Input: part model. Units: mm. Frame: model coordinates. Face numbers are marked on the shaded views. A direction names the side the tool comes from. Give positions to 0.01 mm unless a question says otherwise; leave off trailing zeros. Loops run counter-clockwise (first coordinate to the right, second up) from the corner with the lowest first, then second, coordinate; pieces in that order, holes last. Notation, with made-up numbers: (71, 62.25) -> (76, 62.25) arc R31 cw to (76, 97.25) -> close; hole circle Ø1 at (-2.5, -37.5). An arc over 180 degrees is marked (long way). Use CSV: the item, a comma, the result in double quotes.
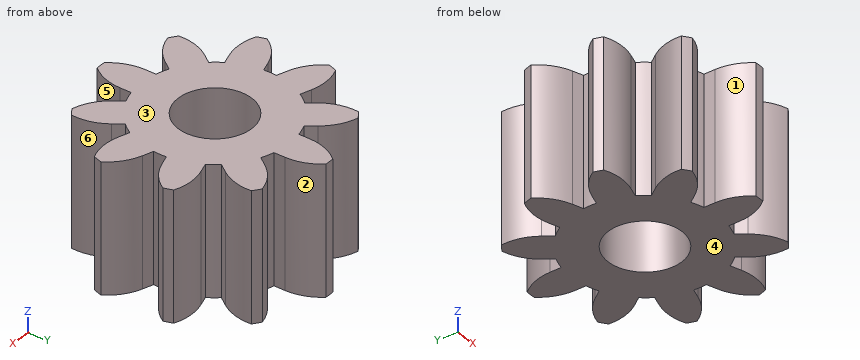
```python
from build123d import *

# Parameters (mm, degrees)
ESBO_O1_R                = 2
RESSALTO_EXTRUS_O1_DEPTH = 3.5
CORTE_EXTRUS_O1_REACH    = 7.574
ESBO_O2_R                = 1


with BuildPart() as part:
    # Esboço1 → Ressalto-extrusão1 (new body)
    with BuildSketch(Plane.XY):
        Circle(ESBO_O1_R)
        with BuildLine():
            Line((-1.99959981, -1.122867364), (-1.714282855, -1.030162265))
            ThreePointArc((-1.714282855, -1.030162265), (-1.902113033, -0.618033989), (-1.99239815, -0.174211401))
            Line((-1.99239815, -0.174211401), (-2.277715105, -0.266916499))
            ThreePointArc((-2.277715105, -0.266916499), (-2.695113044, -0.490735084), (-3.008300145, -0.846023191))
            ThreePointArc((-3.008300145, -0.846023191), (-2.972051613, -0.965678107), (-2.931045896, -1.08378732))
            ThreePointArc((-2.931045896, -1.08378732), (-2.4688391, -1.187134677), (-1.99959981, -1.122867364))
        make_face()
        with BuildLine():
            Line((-2.277715105, 0.266916499), (-1.99239815, 0.174211401))
            ThreePointArc((-1.99239815, 0.174211401), (-1.902113033, 0.618033989), (-1.714282855, 1.030162265))
            Line((-1.714282855, 1.030162265), (-1.99959981, 1.122867364))
            ThreePointArc((-1.99959981, 1.122867364), (-2.4688391, 1.187134677), (-2.931045896, 1.08378732))
            ThreePointArc((-2.931045896, 1.08378732), (-2.972051613, 0.965678107), (-3.008300145, 0.846023191))
            ThreePointArc((-3.008300145, 0.846023191), (-2.695113044, 0.490735084), (-2.277715105, 0.266916499))
        make_face()
        with BuildLine():
            Line((-1.685820646, 1.554747331), (-1.509485071, 1.312042233))
            ThreePointArc((-1.509485071, 1.312042233), (-1.175570505, 1.618033989), (-0.781369776, 1.84104896))
            Line((-0.781369776, 1.84104896), (-0.957705351, 2.083754058))
            ThreePointArc((-0.957705351, 2.083754058), (-1.299552532, 2.411559342), (-1.734231738, 2.599627912))
            ThreePointArc((-1.734231738, 2.599627912), (-1.836828913, 2.528178107), (-1.936485986, 2.452681599))
            ThreePointArc((-1.936485986, 2.452681599), (-1.891945409, 1.981160724), (-1.685820646, 1.554747331))
        make_face()
        with BuildLine():
            Line((-0.45, 2.248717527), (-0.45, 1.948717527))
            ThreePointArc((-0.45, 1.948717527), (0, 2), (0.45, 1.948717527))
            Line((0.45, 1.948717527), (0.45, 2.248717527))
            ThreePointArc((0.45, 2.248717527), (0.366118933, 2.714850303), (0.125, 3.122498999))
            ThreePointArc((0.125, 3.122498999), (0, 3.125), (-0.125, 3.122498999))
            ThreePointArc((-0.125, 3.122498999), (-0.366118933, 2.714850303), (-0.45, 2.248717527))
        make_face()
        with BuildLine():
            ThreePointArc((0.781369776, 1.84104896), (1.175570505, 1.618033989), (1.509485071, 1.312042233))
            Line((1.509485071, 1.312042233), (1.685820646, 1.554747331))
            ThreePointArc((1.685820646, 1.554747331), (1.891945409, 1.981160724), (1.936485986, 2.452681599))
            ThreePointArc((1.936485986, 2.452681599), (1.836828913, 2.528178107), (1.734231738, 2.599627912))
            ThreePointArc((1.734231738, 2.599627912), (1.299552532, 2.411559342), (0.957705351, 2.083754058))
            Line((0.957705351, 2.083754058), (0.781369776, 1.84104896))
        make_face()
        with BuildLine():
            ThreePointArc((1.714282855, 1.030162265), (1.902113033, 0.618033989), (1.99239815, 0.174211401))
            Line((1.99239815, 0.174211401), (2.277715105, 0.266916499))
            ThreePointArc((2.277715105, 0.266916499), (2.695113044, 0.490735084), (3.008300145, 0.846023191))
            ThreePointArc((3.008300145, 0.846023191), (2.972051613, 0.965678107), (2.931045896, 1.08378732))
            ThreePointArc((2.931045896, 1.08378732), (2.4688391, 1.187134677), (1.99959981, 1.122867364))
            Line((1.99959981, 1.122867364), (1.714282855, 1.030162265))
        make_face()
        with BuildLine():
            ThreePointArc((1.99239815, -0.174211401), (1.902113033, -0.618033989), (1.714282855, -1.030162265))
            Line((1.714282855, -1.030162265), (1.99959981, -1.122867364))
            ThreePointArc((1.99959981, -1.122867364), (2.4688391, -1.187134677), (2.931045896, -1.08378732))
            ThreePointArc((2.931045896, -1.08378732), (2.972051613, -0.965678107), (3.008300145, -0.846023191))
            ThreePointArc((3.008300145, -0.846023191), (2.695113044, -0.490735084), (2.277715105, -0.266916499))
            Line((2.277715105, -0.266916499), (1.99239815, -0.174211401))
        make_face()
        with BuildLine():
            ThreePointArc((1.509485071, -1.312042233), (1.175570505, -1.618033989), (0.781369776, -1.84104896))
            Line((0.781369776, -1.84104896), (0.957705351, -2.083754058))
            ThreePointArc((0.957705351, -2.083754058), (1.299552532, -2.411559342), (1.734231738, -2.599627912))
            ThreePointArc((1.734231738, -2.599627912), (1.836828913, -2.528178107), (1.936485986, -2.452681599))
            ThreePointArc((1.936485986, -2.452681599), (1.891945409, -1.981160724), (1.685820646, -1.554747331))
            Line((1.685820646, -1.554747331), (1.509485071, -1.312042233))
        make_face()
        with BuildLine():
            Line((-0.45, -1.948717527), (-0.45, -2.248717527))
            ThreePointArc((-0.45, -2.248717527), (-0.366118933, -2.714850303), (-0.125, -3.122498999))
            ThreePointArc((-0.125, -3.122498999), (0, -3.125), (0.125, -3.122498999))
            ThreePointArc((0.125, -3.122498999), (0.366118933, -2.714850303), (0.45, -2.248717527))
            Line((0.45, -2.248717527), (0.45, -1.948717527))
            ThreePointArc((0.45, -1.948717527), (0, -2), (-0.45, -1.948717527))
        make_face()
        with BuildLine():
            Line((-0.957705351, -2.083754058), (-0.781369776, -1.84104896))
            ThreePointArc((-0.781369776, -1.84104896), (-1.175570505, -1.618033989), (-1.509485071, -1.312042233))
            Line((-1.509485071, -1.312042233), (-1.685820646, -1.554747331))
            ThreePointArc((-1.685820646, -1.554747331), (-1.891945409, -1.981160724), (-1.936485986, -2.452681599))
            ThreePointArc((-1.936485986, -2.452681599), (-1.836828913, -2.528178107), (-1.734231738, -2.599627912))
            ThreePointArc((-1.734231738, -2.599627912), (-1.299552532, -2.411559342), (-0.957705351, -2.083754058))
        make_face()
    extrude(amount=RESSALTO_EXTRUS_O1_DEPTH)

    # Esboço2 → Corte-extrusão1 (cut, up to next)
    with BuildSketch(Plane.XY.offset(3.5), mode=Mode.PRIVATE) as corte_extrus_o1_sk1:
        Circle(ESBO_O2_R)
    corte_extrus_o1_tool1 = extrude(corte_extrus_o1_sk1.sketch, amount=-CORTE_EXTRUS_O1_REACH, mode=Mode.PRIVATE) & part.part
    add(corte_extrus_o1_tool1.solids().sort_by_distance((0, 0, 3.5))[0], mode=Mode.SUBTRACT)


solid = part.part
```
1) Section query B-B (x = 0). Return loops of the section in (y, z) (3 decimals), then the cut area to 3 significant figures.
From the geometry:
outline,"(-3.125, 0) -> (-1, 0) -> (-1, 3.5) -> (-3.125, 3.5) -> close; (1, 0) -> (3.125, 0) -> (3.125, 3.5) -> (1, 3.5) -> close"
area,"14.9 mm^2"
2) Section query A-A (y = 0). Return loops of the section in (x, z).
From the geometry:
outline,"(-2, 0) -> (-1, 0) -> (-1, 3.5) -> (-2, 3.5) -> close; (1, 0) -> (2, 0) -> (2, 3.5) -> (1, 3.5) -> close"
3) Reachability of the marked faces 1, 2 and 3 from +Z, -Z, +X, -X, +Y, -Y: full face, straight path, thin tool, end or side. Return the list, or none.
From the geometry:
face 1,"+Z, -Z, -Y"
face 2,"+Z, -Z, +Y"
face 3,"+Z, +X, -X, +Y, -Y"
4) Ray query, line 1 (X direction, y = 2.5, z = 2.8) (3 decimals); line 2 (Y direction, x = 0, z = 0.85) (3 decimals); line 3 (Y direction, x = -1.75, z = 3.3). Return the intervals inside material, ascending.
From the geometry:
line 1,"x = -1.875 to -1.454, -0.426 to 0.426, 1.454 to 1.875"
line 2,"y = -3.125 to -1, 1 to 3.125"
line 3,"y = -2.59 to -1.65, -1.04 to 1.04, 1.65 to 2.59"
5) Mould query, pull axis X, two halves, no side actions, for the marked faces 4, 5 and 6. Classes: pulls with the +X half, pulls with the -X half, needs draft (parallel to the pull), parting line crosses it, or undercut.
From the geometry:
face 4,"needs draft"
face 5,"undercut"
face 6,"pulls with the +X half"
6) Section query C-C (y = 2.75). Return loops of the section in (x, z), then the cut area to 3 significant figures.
From the geometry:
outline,"(-0.35, 0) -> (0.35, 0) -> (0.35, 3.5) -> (-0.35, 3.5) -> close"
area,"2.47 mm^2"
7) Contact query for flat-ended pins moving along their axis: pin 1 (1.6 mm diameter, centred on x = 0, y = 0, fed in from -Z); pin 2 (1 mm diameter, centred on x = 1, z = 3, fed in from -Y); pin 3 (2 mm diameter, centred on y = 2, z = 1.5, fed in from +X); pin 4 (2 mm diameter, centred on y = 2, z = 3, fed in from -X). Output: stop coordinate, or through.
From the geometry:
pin 1,"passes through"
pin 2,"stops at y = -2.52"
pin 3,"stops at x = 2.96"
pin 4,"stops at x = -2.96"
